Verification items for this drawing (mm, ordinates from the low corner). Round coordinates to 2 decimals unless told otherwise and drop trailing zeros. Write each loop counter-clockwise with the first axis right and the second up, starting at its lowest first coordinate (ties: lowest second). Pieces come first, ordered by that corner, then holes. Notation, with made-up numbers: (-33.75, 58) - (-12.75, 58) arc R7 ccw to (-12.75, 65) - close; hole circle Ø6 at (83.25, -3.5). An arc over 180 degrees is marked (long way). One line per question, with ' | ' between items. Start each with the question number.
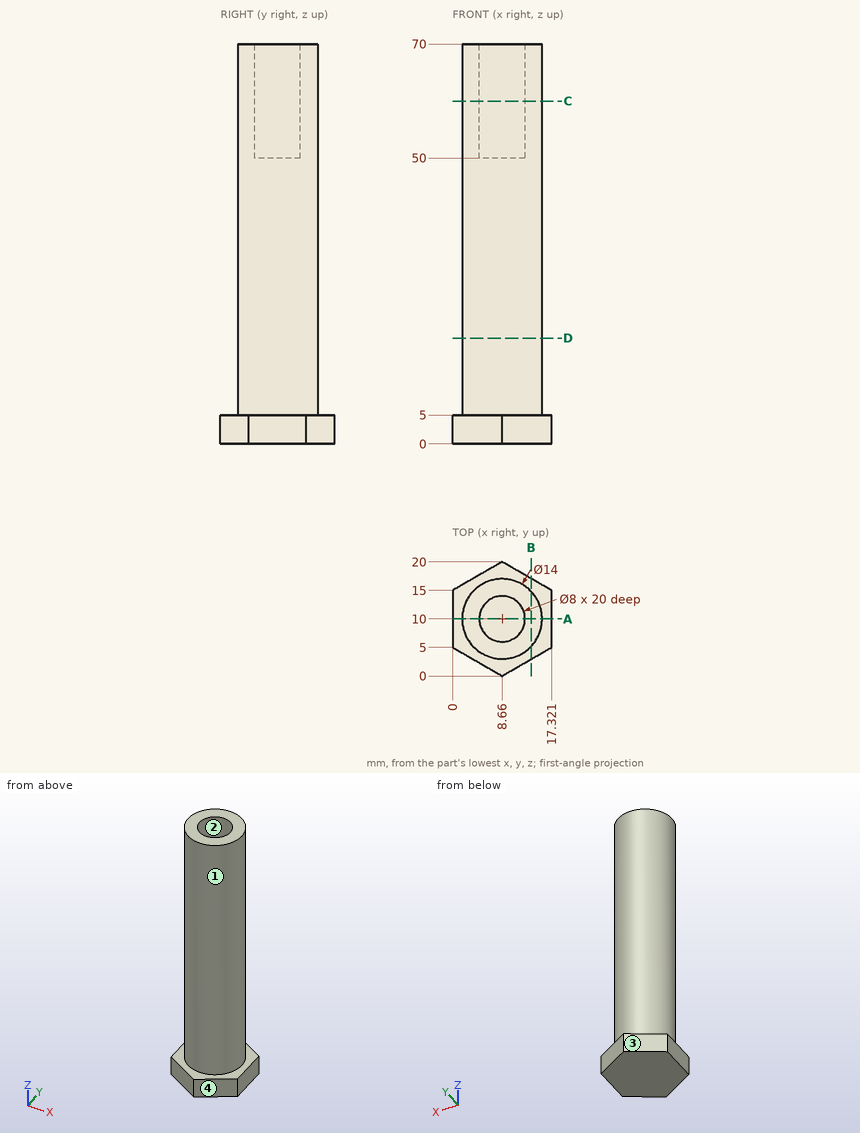
Q1. Go/stop test with flat-tipped pins: P1, Ø8, axis at y = 11.5, z = 45.5, coming from the -X side; P2, Ø4, axis at x = 10, y = 10, coming from the +Z side; P3, Ø8, axis at y = 15, z = 60, coming from the +X side; P4, Ø7, axis at x = 8.66, y = 10, coming from the -Z side. Record where each tip stops, or that it passes through.
Q2. Section check C-C, the plane z = 60. Record the cut outline in (x, y).
Q3. Section check A-A, the plane y = 10. Record the cut outline in (x, z).
Q4. Section check D-D, the plane z = 18.5. Record the cut outline in (x, y).
Q5. Thickness scan on line 1 (Z direction, x = 8.25, y = 6.5); line 2 (Z direction, x = 11, y = 3.25); line 3 (X direction, y = 10.25, z = 5.5) (1 decimal). Record the ranges inside material, lowest first.
Q6. Draft check along X on the marked faces 1, 2, 3 and 4. Enter one of: pulls with the +X half, pulls with the -X half, needs draft (parallel to the pull), parting line crosses it, or undercut.
Q7. Section check B-B, the plane x = 13.75. Record the cut outline in (y, z) (1 decimal).
Result sheet:
1) P1: x = 1.66 | P2: z = 50 | P3: x = 15.59 | P4: z = 0
2) outline: circle Ø14 at (8.66, 10); hole circle Ø8 at (8.66, 10)
3) outline: (0, 0) - (17.32, 0) - (17.32, 5) - (15.66, 5) - (15.66, 70) - (12.66, 70) - (12.66, 50) - (4.66, 50) - (4.66, 70) - (1.66, 70) - (1.66, 5) - (0, 5) - close
4) outline: circle Ø14 at (8.66, 10)
5) line 1: 0 to 50 | line 2: 0 to 5 | line 3: 1.7 to 15.7
6) face 1: parting line crosses it | face 2: undercut | face 3: pulls with the -X half | face 4: pulls with the +X half
7) outline: (2.9, 0) - (17.1, 0) - (17.1, 5) - (14.8, 5) - (14.8, 70) - (5.2, 70) - (5.2, 5) - (2.9, 5) - close
